Could you check a few things on this drawing? It's one solid part, dimensions in mm from its lowest x, y, z. Give positions to 0.01 mm unless a question says otherwise; leave off trailing zeros. Order: outer loops, then holes, each group sorted by start corner. A loop starts at its lowest first (then second) coordinate and runs counter-clockwise, first axis right, second up. Notation, with made-up numbers: M 55.5,-6.5 L 77.5,-6.5 A22 ccw 77.5,16.5 Z; hole C -10,28 d1. An arc over 180 degrees is marked long. One line per item, written item: value. Start each with the question number.
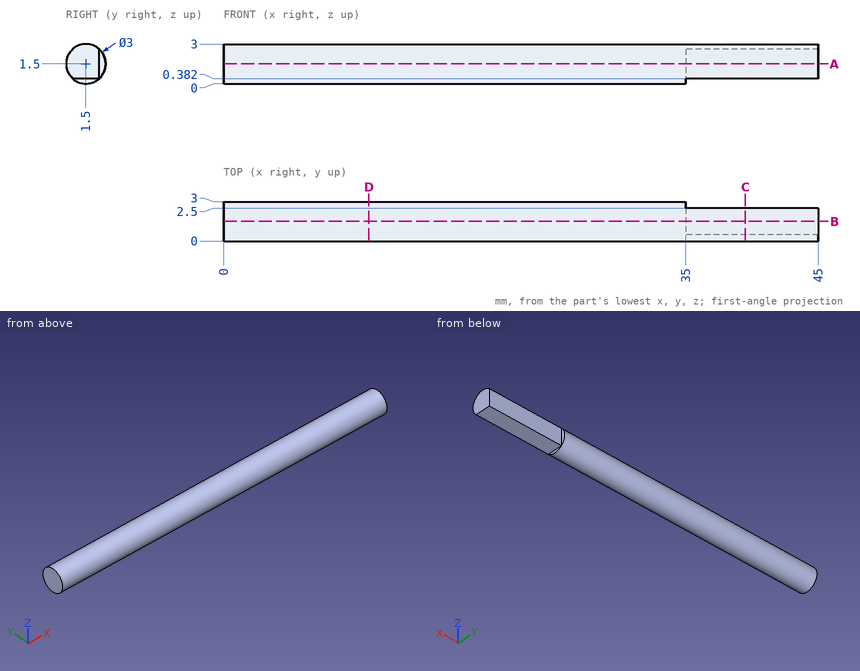
Item 1: Please list where these lines run through material, in increasing order: probe 1 along Y at (x, z) = (11, 2.5); probe 2 along Y at (x, z) = (34, 1.6); probe 3 along Z at (x, y) = (27.5, 0.35). Write a range as [from, to].
Item 2: Will this pin go through, and if not, where does the flat tip stop? P1, Ø1.6, axis at x = 38.5, y = 1, coming from the -Z side.
Item 3: I want a section at D-D on x = 11. Write out the boundary of the cut face in (y, z), plus the area to 3 significant figures.
Item 4: I want a section at C-C on x = 39.5. Write out the boundary of the cut face in (y, z), plus the area to 3 significant figures.
Item 5: I want a section at A-A on z = 1.5. Write out the boundary of the cut face in (x, y), plus the area to 3 significant figures.
Item 6: I want a section at B-B on y = 1.5. Write out the boundary of the cut face in (x, z), plus the area to 3 significant figures.
Answer below:
1. probe 1: y = [0.38, 2.62]
1. probe 2: y = [0, 3]
1. probe 3: z = [0.54, 2.46]
2. P1: stops at z = 0.38
3. outline: C 1.5,1.5 d3
3. area: 7.07 mm²
4. outline: M 0.5,0.38 L 2.5,0.38 L 2.5,2.62 A1.5 ccw Z
4. area: 5.77 mm²
5. outline: M 0,0 L 45,0 L 45,2.5 L 35,2.5 L 35,3 L 0,3 Z
5. area: 130 mm²
6. outline: M 0,0 L 35,0 L 35,0.38 L 45,0.38 L 45,3 L 0,3 Z
6. area: 131 mm²
